Could you check a few things on this drawing? It's one solid part, dimensions in mm from its lowest x, y, z. A direction names the side the tool comes from. Round coordinates to 2 decimals unless told otherwise and drop trailing zeros. Answer as CSV lines item,"result".
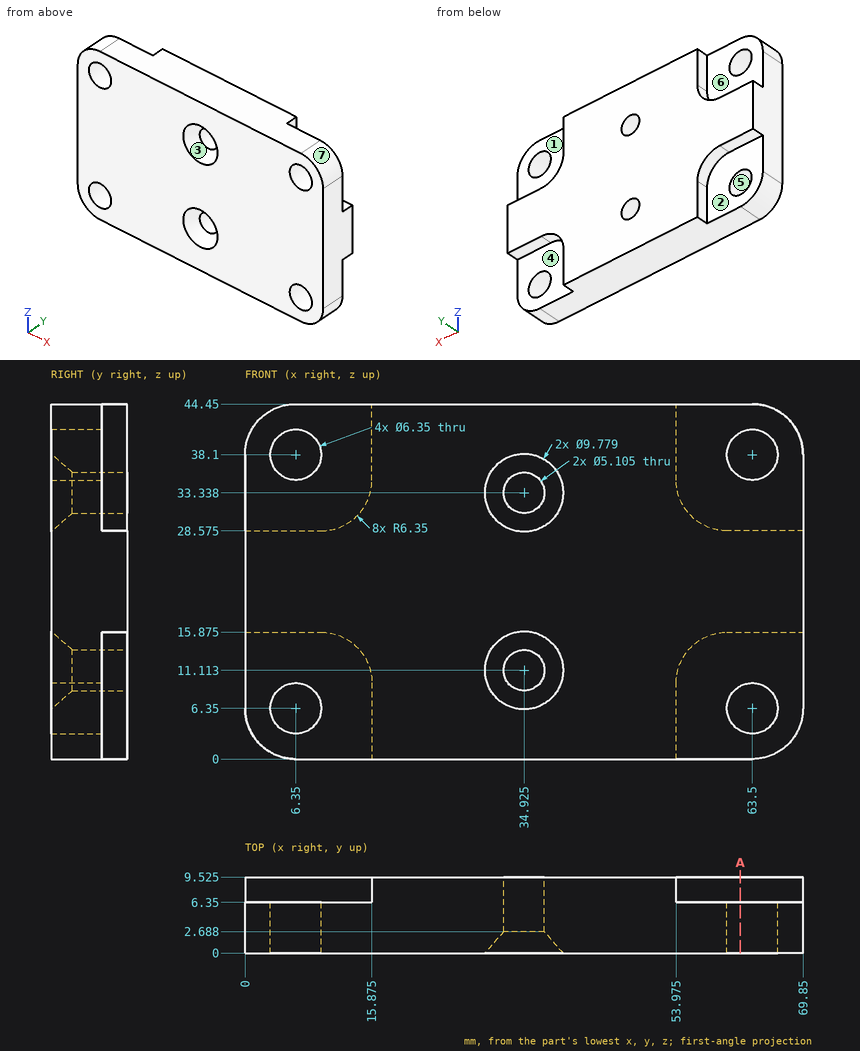
1. For pin 1 Ø6 at (x, z) = (34.92, 11.11) entering from -Y (1 decimal); pin 2 Ø17.5 at (x, z) = (4.5, 5) entering from +Y; pin 3 Ø8.5 at (x, z) = (63.5, 6.35) entering from +Y; pin 4 Ø5.5 at (x, z) = (6.35, 38.1) entering from -Y, each with a flat end and sliding along its axis, tell me the tip position at first contact or that it passes through.
Numbers:
pin 1,"stops at y = 2.2"
pin 2,"stops at y = 6.35"
pin 3,"stops at y = 6.35"
pin 4,"passes through"
2. If I drill on line 1 (X direction, y = 5, z = 40.5); line 2 (X direction, y = 7.5, z = 42.5) (1 decimal); line 3 (Y direction, x = 60.5, z = 30), over which ranges is the centre line in solid material (lowest first)?
Numbers:
line 1,"x = 0.47 to 4.27, 8.43 to 61.42, 65.58 to 69.38"
line 2,"x = 15.9 to 54"
line 3,"y = 0 to 6.35"
3. If we mould it in two halves opening along X, with no side actions, what happens to the marked faces 5, 6 and 7? For each: released by +X, released by -X, zero draft, split by the parting line, or undercut.
Numbers:
face 5,"undercut"
face 6,"zero draft"
face 7,"released by +X"
4. On a 3-axis mill with a long thin cutter (end or side, diameter ignored), from which of +Z, -Z, +X, -X, +Y, -Y can I reach the whole of each face in a straight line? I mean the marked faces 1, 2, 3 and 4. Say none if no direction works.
Numbers:
face 1,"+Z, +X, +Y"
face 2,"-Z, -X, +Y"
face 3,"-Y"
face 4,"-Z, +X, +Y"
5. Suppose I cut it at A-A on x = 62. Count the separate pieces of the cut face and the enclosed holes in it.
Numbers:
separate pieces,"3"
enclosed holes,"0"
